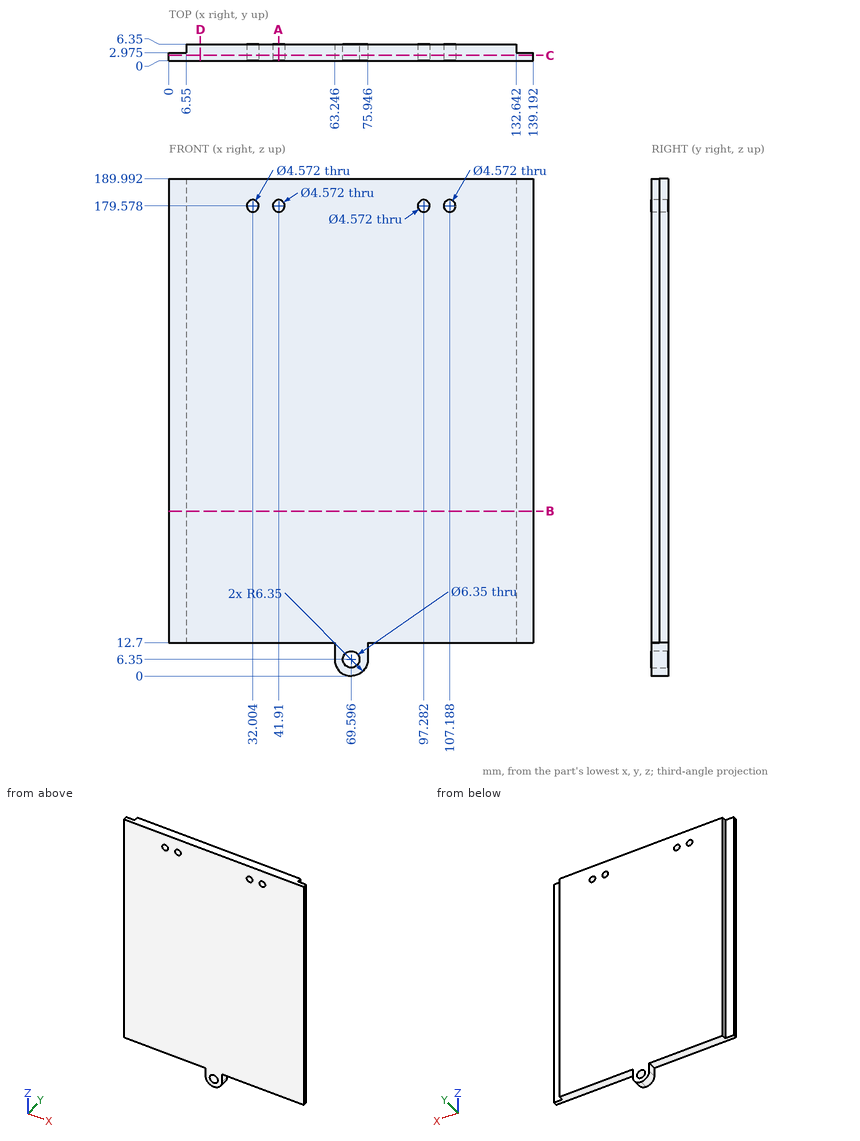
Here's the drawing with two shaded views (mm, measured from the low corner). I have some questions. Give positions to 0.01 mm unless a question says otherwise; leave off trailing zeros. Order: outer loops, then holes, each group sorted by start corner. A loop starts at its lowest first (then second) coordinate and runs counter-clockwise, first axis right, second up. Notation, with made-up numbers: M -13,8.25 L -7,8.25 A33 cw -7,41.25 Z; hole C 13.5,-27 d10. An arc over 180 degrees is marked long. Answer as a JSON object with one key per item and string values. Group by question number.
1) Suppose I cut it at D-D, the plane x = 12. Write out the boundary of the cut face in (y, z), plus the area to 3 significant figures.
2) Suppose I cut it at C-C, the plane y = 2. Count the separate pieces of the cut face and the enclosed holes in it, plus the area to 3 significant figures.
3) I'm going to push flat-ended pins straight in: pin 1 Ø1 at (y, z) = (4, 96.5) entering from +X; pin 2 Ø1.9 at (y, z) = (3, 9.5) entering from -X; pin 3 Ø1 at (y, z) = (5.5, 111.5) entering from -X. Where does each tip first touch, or does it pass through?
4) Suppose I cut it at A-A, the plane x = 41.91. Write out the boundary of the cut face in (y, z).
5) Please list where these lines run through material, in increasing order: L1, parallel to X at y = 4.25, z = 179.5; L2, parallel to Z at x = 70, y = 0.75; L3, parallel to Z at x = 129, y = 3.5. Write a range as [from, to].
6) Suppose I cut it at B-B, the plane z = 63. Write out the boundary of the cut face in (x, y) (3 decimals).
Results found:
{
 "1": {"outline": "M 0,12.7 L 6.35,12.7 L 6.35,189.99 L 0,189.99 Z", "area": "1,130 mm²"},
 "2": {"separate pieces": "1", "enclosed holes": "5", "area": "24,700 mm²"},
 "3": {"pin 1": "x = 132.64", "pin 2": "x = 63.25", "pin 3": "x = 6.55"},
 "4": {"outline": "M 0,12.7 L 6.35,12.7 L 6.35,177.29 L 0,177.29 Z; M 0,181.86 L 6.35,181.86 L 6.35,189.99 L 0,189.99 Z"},
 "5": {"L1": "[6.55, 29.72], [34.29, 39.63], [44.19, 95], [99.57, 104.9], [109.47, 132.64]", "L2": "[0.01, 3.2], [9.5, 189.99]", "L3": "[12.7, 189.99]"},
 "6": {"outline": "M 0,0 L 139.192,0 L 139.192,2.975 L 132.642,2.975 L 132.642,6.35 L 6.55,6.35 L 6.55,2.975 L 0,2.975 Z"}
}
